from build123d import *

# Parameters (mm, degrees)
F0_R     = 1.75
F0_W     = 14
F0_H     = 5
F0_W_2   = 5
F0_H_2   = 11
F0_R_2   = 3.5
F1_DEPTH = 6
F2_DEPTH = 2
F4_DEPTH = 3
F5_R     = 5


with BuildPart() as f1:
    # F0 (on Front) → F1 (new body)
    with BuildSketch(Plane.XZ):
        Polygon((-22, -20), (22, -20), (22, 20), (2, 20), (2, -3.5), (-22, -3.5), align=None)
        with Locations((-18.5, -16)):
            Circle(F0_R, mode=Mode.SUBTRACT)
        with Locations((-9, -10)):
            Rectangle(F0_W, F0_H, mode=Mode.SUBTRACT)
        with Locations((0.5, -16)):
            Circle(F0_R, mode=Mode.SUBTRACT)
        with Locations((6.5, -10.5)):
            Rectangle(F0_W_2, F0_H_2, mode=Mode.SUBTRACT)
        with Locations((12, 1.5)):
            Circle(F0_R_2, mode=Mode.SUBTRACT)
        with Locations((12, 13.5)):
            Circle(F0_R_2, mode=Mode.SUBTRACT)
        with Locations((-9, -10)):
            Rectangle(F0_W, F0_H)
        with Locations((6.5, -10.5)):
            Rectangle(F0_W_2, F0_H_2)
        with Locations((12, 1.5)):
            Circle(F0_R_2)
        with Locations((12, 1.5)):
            Circle(F0_R, mode=Mode.SUBTRACT)
        with Locations((12, 13.5)):
            Circle(F0_R_2)
        with Locations((12, 13.5)):
            Circle(F0_R, mode=Mode.SUBTRACT)
    extrude(amount=-F1_DEPTH)

    # F0 (on Front) → F2 (cut)
    with BuildSketch(Plane.XZ):
        with Locations((6.5, -10.5)):
            Rectangle(F0_W_2, F0_H_2)
        with Locations((-9, -10)):
            Rectangle(F0_W, F0_H)
        with Locations((12, 13.5)):
            Circle(F0_R_2)
        with Locations((12, 13.5)):
            Circle(F0_R, mode=Mode.SUBTRACT)
        with Locations((12, 1.5)):
            Circle(F0_R_2)
        with Locations((12, 1.5)):
            Circle(F0_R, mode=Mode.SUBTRACT)
    extrude(amount=-F2_DEPTH, mode=Mode.SUBTRACT)

    # F3 (on face) → F4 (cut)
    with BuildSketch(Plane(origin=(0, 6, 0), x_dir=(-1, 0, 0), z_dir=(0, 1, 0))):
        Polygon((-0.5, -12.535898), (-3.5, -14.267949), (-3.5, -17.732051), (-0.5, -19.464102), (2.5, -17.732051), (2.5, -14.267949), align=None)
        Polygon((15.5, -14.267949), (15.5, -17.732051), (18.5, -19.464102), (21.5, -17.732051), (21.5, -14.267949), (18.5, -12.535898), align=None)
    extrude(amount=-F4_DEPTH, mode=Mode.SUBTRACT)

    # F5
    f5_edges = [f1.edges().sort_by_distance(p)[0] for p in [
        (2, 3, -3.5),
        (2, 3, 20),
        (22, 3, 20),
    ]]
    fillet(f5_edges, radius=F5_R)


solid = f1.part
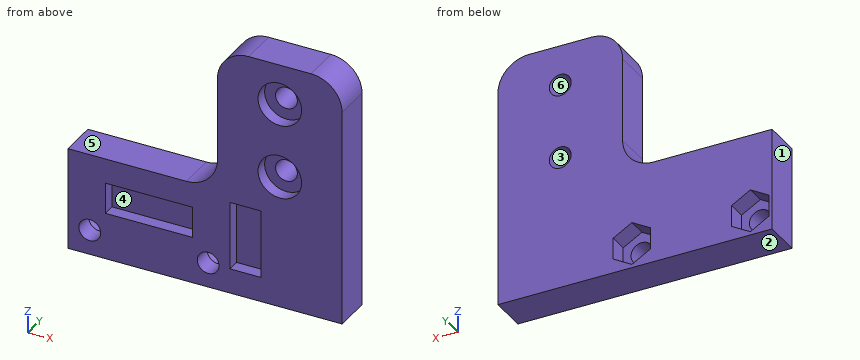
Verification items for the finished model (mm, model axes). Face numbers are marked on the shaded views. A direction names the side the tool comes from. Give positions to 0.01 mm unless a question says otherwise; leave off trailing zeros. Write each loop counter-clockwise with the first axis right and the second up, starting at its lowest first coordinate (ties: lowest second). Pieces come first, ordered by that corner, then holes.
(1) Cross-section at A-A (z = 13.5). Enter the section's corners in (x, y).
(2) Mould release check, pull along X, two halves, no side actions. Record for the marked faces 1, 2 and 3: +X half, -X half, draft (parallel to the pull), parting line (faces both ways), or undercut.
(3) Cross-section at B-B (x = 12). Enter the section's corners in (y, z), plus the area to 3 significant figures.
(4) Cross-section at D-D (z = -9.5). Enter the section's corners in (x, y), plus the area to 3 significant figures.
(5) Gauge pin test, flat ends, axial feed: pin 1 (1.8 mm diameter, centred on x = -19.5, z = -15.5, fed in from +Y); pin 2 (1.6 mm diameter, centred on x = -11.5, y = 0.5, fed in from +Z); pin 3 (2.5 mm diameter, centred on x = 7.5, z = -10, fed in from -Y); pin 4 (1 mm diameter, centred on x = 12, z = 2, fed in from -Y). Record the tip position at first contact, or that the pin passes through.
(6) Access from +Z, -Z, +X, -X, +Y, -Y to the whole of each face (thin tool, end or side, straight path). Record for the marked faces 4, 5 and 6.
(7) Material ranges on line 1 (Z direction, x = 12, y = 2.8); line 2 (X direction, y = 4.55, z = -15); line 3 (Z direction, x = 12, y = 0.8), recorded low to high.
(8) Cross-section at C-C (y = 3.5). Enter the section's corners in (x, z), plus the area to 3 significant figures.
Worked out:
1. outline: (2, 0) - (8.5, 0) - (8.5, 2) - (10.25, 2) - (10.25, 6) - (2, 6) - close; (13.75, 2) - (15.5, 2) - (15.5, 0) - (22, 0) - (22, 6) - (13.75, 6) - close
2. face 1: -X half
2. face 2: draft
2. face 3: undercut
3. outline: (0, -20) - (6, -20) - (6, -0.25) - (2, -0.25) - (2, -2) - (0, -2) - close; (0, 5) - (2, 5) - (2, 3.25) - (6, 3.25) - (6, 11.75) - (2, 11.75) - (2, 10) - (0, 10) - close; (0, 17) - (2, 17) - (2, 15.25) - (6, 15.25) - (6, 20) - (0, 20) - close
3. area: 184 mm2
4. outline: (-22, 0) - (-16, 0) - (-16, 2) - (-2, 2) - (-2, 0) - (4, 0) - (4, 2) - (9, 2) - (9, 0) - (22, 0) - (22, 6) - (-22, 6) - close
4. area: 226 mm2
5. pin 1: stops at y = 3
5. pin 2: stops at z = -3.5
5. pin 3: stops at y = 2
5. pin 4: passes through
6. face 4: -Y
6. face 5: +Z, -X, +Y, -Y
6. face 6: +Y, -Y
7. line 1: z = -20 to -0.25, 3.25 to 11.75, 15.25 to 20
7. line 2: x = -22 to -21.5, -15.5 to -2.5, 3.5 to 22
7. line 3: z = -20 to -2, 5 to 10, 17 to 20
8. outline: (-22, -20) - (22, -20) - (22, 15) arc R5 ccw to (17, 20) - (7, 20) arc R5 ccw to (2, 15) - (2, 1.5) arc R5 cw to (-3, -3.5) - (-22, -3.5) - close; hole (-21.5, -17.73) - (-18.5, -19.46) - (-15.5, -17.73) - (-15.5, -14.27) - (-18.5, -12.54) - (-21.5, -14.27) - close; hole (-2.5, -17.73) - (0.5, -19.46) - (3.5, -17.73) - (3.5, -14.27) - (0.5, -12.54) - (-2.5, -14.27) - close; hole circle Ø3.5 at (12, 1.5); hole circle Ø3.5 at (12, 13.5)
8. area: 1,110 mm2
